Input: part model. Units: mm. Frame: model coordinates. Face numbers are marked on the shaded views. A direction names the side the tool comes from. Give positions to 0.01 mm unless a question says otherwise; leave off trailing zeros. Loops run counter-clockwise (first coordinate to the right, second up) from the corner with the lowest first, then second, coordinate; pieces in that order, holes last. Notation, with made-up numbers: M 3,13.5 L 53,13.5 A24 ccw 53,35.5 Z; hole C -1,-38 d2. An arc over 180 degrees is marked long. Use CSV: the item, a comma, the result in double quotes. Start each with the question number.
Q1. Reachability of the marked faces 4, 5, 6, 7 and 8 from +Z, -Z, +X, -X, +Y, -Y: full face, straight path, thin tool, end or side. Return the list, or none.
Q2. Section D-D, the plane z = 54.5. Output: boundary loops of the cut face in (x, y).
Q3. Pull-direction query (Y, two-part tool) for the marked faces 1, 2 and 3; classes: released by +Y, released by -Y, zero draft, split by the parting line, or undercut.
Q4. Material intervals for line 1 along Y through (x, z) = (135.5, 44); line 2 along Z through (x, y) = (322, 87); line 3 along X through (y, z) = (624, 34), sorted ascending.
Q5. Section A-A, the plane z = 650.5. Output: boundary loops of the cut face in (x, y).
Q6. Section C-C, the plane z = 138.5. Output: boundary loops of the cut face in (x, y), plus the area to 3 significant figures.
Q7. Pin query (flat end, axial travel): pin 1 (5.5 mm diameter, centred on x = 446.5, z = 413, fed in from -Y); pin 2 (5 mm diameter, centred on y = 100, z = 216, fed in from -X); pin 3 (14.5 mm diameter, centred on x = 450, z = 561, fed in from +Y); pin 4 (6 mm diameter, centred on y = 76, z = 760, fed in from -X). Return the tip coordinate at first contact, or that it passes through.
Q8. Section B-B, the plane y = 178. Output: boundary loops of the cut face in (x, z).
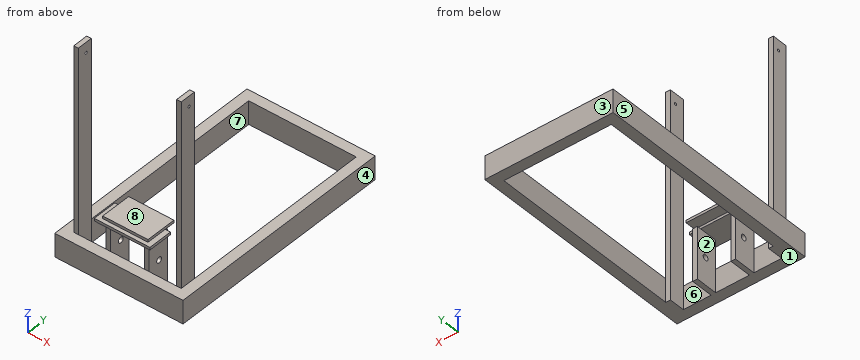
from build123d import *

# Parameters (mm, degrees)
F0_W      = 495.3
F0_H      = 890
F0_W_2    = 415.3
F0_H_2    = 810
F1_DEPTH  = 90
F2_W      = 17.5
F2_H      = 85
F2_W_2    = 18
F3_DEPTH  = 200
F4_W      = 17.5
F4_H      = 60
F4_W_2    = 18
F5_DEPTH  = 800
F6_R      = 5
F7_DEPTH  = 453
F8_R      = 11.1125
F9_DEPTH  = 184
F10_W     = 215
F10_H     = 95
F11_DEPTH = 10
F12_W     = 175
F12_H     = 80
F12_H_2   = 40
F13_DEPTH = 10


with BuildPart() as f1:
    # F0 (on Top) → F1 (new body)
    with BuildSketch(Plane.XY):
        with Locations((247.65, 445)):
            Rectangle(F0_W, F0_H)
        with Locations((247.65, 445)):
            Rectangle(F0_W_2, F0_H_2, mode=Mode.SUBTRACT)
    extrude(amount=F1_DEPTH)

    # F2 (on Top) → F3 (join)
    with BuildSketch(Plane.XY):
        with Locations((173.75, 82.5)):
            Rectangle(F2_W, F2_H)
        with Locations((321.3, 82.5)):
            Rectangle(F2_W_2, F2_H)
    extrude(amount=F3_DEPTH)

    # F4 (on Top) → F5 (join)
    with BuildSketch(Plane.XY):
        with Locations((48.75, 70)):
            Rectangle(F4_W, F4_H)
        with Locations((446.3, 70)):
            Rectangle(F4_W_2, F4_H)
    extrude(amount=F5_DEPTH)

    # F6 (on face) → F7 (cut)
    with BuildSketch(Plane(origin=(40, 0, 0), x_dir=(0, -1, 0), z_dir=(-1, 0, 0))):
        with Locations((-76, 760)):
            Circle(F6_R)
    extrude(amount=-F7_DEPTH, mode=Mode.SUBTRACT)

    # F8 (on face) → F9 (cut)
    with BuildSketch(Plane(origin=(165, 0, 0), x_dir=(0, -1, 0), z_dir=(-1, 0, 0))):
        with Locations((-87, 105)):
            Circle(F8_R)
    extrude(amount=-F9_DEPTH, mode=Mode.SUBTRACT)

    # F10 (on face) → F11 (join)
    with BuildSketch(Plane.XY.offset(200)):
        with Locations((247.5, 62.5)):
            Rectangle(F10_W, F10_H)
    extrude(amount=F11_DEPTH)

    # F12 (on face) → F13 (join)
    with BuildSketch(Plane.XY.offset(210)):
        with Locations((247.5, 70)):
            Rectangle(F12_W, F12_H)
        with Locations((247.5, 130)):
            Rectangle(F12_W, F12_H_2)
    extrude(amount=F13_DEPTH)


solid = f1.part
A:
1,face 4,"+Z, -Z, +X, +Y, -Y"
1,face 5,"+Z, -Z, -X, +Y, -Y"
1,face 6,"-Z"
1,face 7,"+Z, -Z"
1,face 8,"+Z, +Y, -Y"
2,outline,"M 0,0 L 495.3,0 L 495.3,890 L 0,890 Z; hole M 40,100 L 57.5,100 L 57.5,40 L 165,40 L 165,125 L 182.5,125 L 182.5,40 L 312.3,40 L 312.3,125 L 330.3,125 L 330.3,40 L 437.3,40 L 437.3,100 L 455.3,100 L 455.3,850 L 40,850 Z"
3,face 1,"zero draft"
3,face 2,"undercut"
3,face 3,"released by +Y"
4,line 1,"0 to 40, 850 to 890"
4,line 2,"0 to 93.89, 116.11 to 220"
4,line 3,"0 to 40, 455.3 to 495.3"
5,outline,"M 40,40 L 57.5,40 L 57.5,100 L 40,100 Z; M 437.3,40 L 455.3,40 L 455.3,100 L 437.3,100 Z"
6,outline,"M 40,40 L 57.5,40 L 57.5,100 L 40,100 Z; M 165,40 L 182.5,40 L 182.5,125 L 165,125 Z; M 312.3,40 L 330.3,40 L 330.3,125 L 312.3,125 Z; M 437.3,40 L 455.3,40 L 455.3,100 L 437.3,100 Z"
6,area,"5,150 mm^2"
7,pin 1,"y = 40"
7,pin 2,"x = 40"
7,pin 3,"y = 100"
7,pin 4,"through"
8,outline,"M 0,0 L 40,0 L 40,90 L 0,90 Z; M 455.3,0 L 495.3,0 L 495.3,90 L 455.3,90 Z"
